The model under review builds one solid part; all positions refer to its coordinate system, in mm. Face numbers are marked on the shaded views. Coordinates: 2 decimals unless noted, no trailing zeros. Order: outer loops, then holes, each group sorted by start corner. A loop starts at its lowest first (then second) coordinate and runs counter-clockwise, first axis right, second up. Notation, with made-up numbers: M -9,79.5 L 26,79.5 A25 ccw 26,103.5 Z; hole C 20,1 d5. An arc over 180 degrees is marked long. Write each question's results on one line, items separated by ' | '.
from build123d import *

# Parameters (mm, degrees)
SKETCH_1_R          = 20
EXTRUDE_1_DEPTH     = 14
SKETCH_2_R          = 31.5
EXTRUDE_2_DEPTH     = 151
SKETCH_1_3_R        = 20
CUT_EXTRUDE_1_DEPTH = 175.982394882


with BuildPart() as part:
    # Sketch 1 → Extrude 1 (new body)
    with BuildSketch(Plane.XY):
        with BuildLine():
            Line((-35.09399548, 30.506744848), (-35.09399548, -30.506744848))
            ThreePointArc((-35.09399548, -30.506744848), (0, -46.5), (35.09399548, -30.506744848))
            Line((35.09399548, -30.506744848), (35.09399548, 30.506744848))
            ThreePointArc((35.09399548, 30.506744848), (0, 46.5), (-35.09399548, 30.506744848))
        make_face()
        Circle(SKETCH_1_R, mode=Mode.SUBTRACT)
    extrude(amount=-EXTRUDE_1_DEPTH)

    # Sketch 2 → Extrude 2 (add)
    with BuildSketch(Plane(origin=(0, 0, -14), x_dir=(-1, 0, 0), z_dir=(0, 0, -1))):
        Circle(SKETCH_2_R)
    extrude(amount=EXTRUDE_2_DEPTH)

    # Sketch 1_3 → Cut-Extrude 1 (cut, through all)
    with BuildSketch(Plane.XY):
        Circle(SKETCH_1_3_R)
    extrude(amount=-CUT_EXTRUDE_1_DEPTH, mode=Mode.SUBTRACT)


solid = part.part
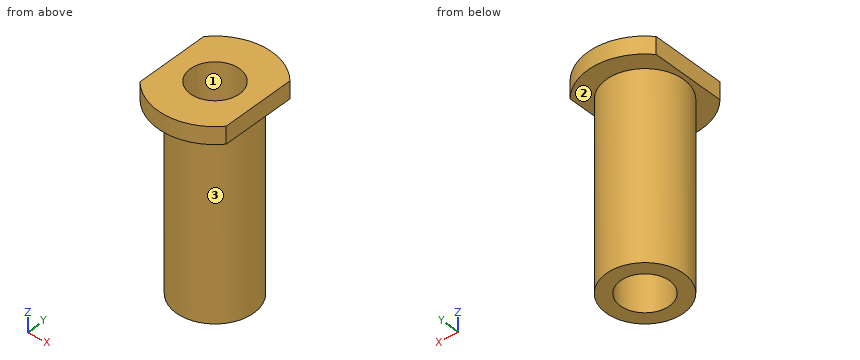
1) The part is to be moulded in two halves that separate along X. For the marked faces 1, 2 and 3, say which applies: pulls with the +X half, pulls with the -X half, needs draft (parallel to the pull), parting line crosses it, or undercut.
Solutions:
face 1: undercut | face 2: needs draft | face 3: parting line crosses it
2) To check wall thickness, follow line 1 along Y through (x, z) = (0, -118); line 2 along Z through (x, y) = (29, 29); line 3 along X through (y, z) = (16, -130). State the ranges of each line that lie inside material, in increasing order.
Solutions:
line 1: -31.5 to -20, 20 to 31.5 | line 2: -14 to 0 | line 3: -27.13 to -12, 12 to 27.13
3) For pin 1 (6 mm diameter, centred on x = 24.5, y = -27, fed in from -Z); pin 2 (1 mm diameter, centred on x = 25, z = -75, fed in from +Y); pin 3 (5 mm diameter, centred on x = -25, z = -37.5, fed in from +Y), all flat-tipped, find the tip position at first contact; note any pin that passes through.
Solutions:
pin 1: z = -14 | pin 2: y = 19.8 | pin 3: y = 22.05
4) Take a section at A-A on y = 0. State the section outline as (x, z) points, plus the area to 3 significant figures.
Solutions:
outline: M -35.09,-14 L -31.5,-14 L -31.5,-165 L -20,-165 L -20,0 L -35.09,0 Z; M 20,-165 L 31.5,-165 L 31.5,-14 L 35.09,-14 L 35.09,0 L 20,0 Z | area: 3,900 mm2
5) Take a section at B-B on x = -12. State the section outline as (y, z) points.
Solutions:
outline: M -44.92,-14 L -29.12,-14 L -29.12,-165 L -16,-165 L -16,0 L -44.92,0 Z; M 16,-165 L 29.12,-165 L 29.12,-14 L 44.92,-14 L 44.92,0 L 16,0 Z
6) Take a section at C-C on z = -103. State the section outline as (x, y) points.
Solutions:
outline: C 0,0 d63; hole C 0,0 d40
7) Take a section at D-D on y = -39.5. State the section outline as (x, z) points, plus the area to 3 significant figures.
Solutions:
outline: M -24.54,-14 L 24.54,-14 L 24.54,0 L -24.54,0 Z | area: 687 mm2
